Work out the finished part from the listing and answer in its coordinate system (mm). A direction names the side the tool comes from. Coordinates: 2 decimals unless noted, no trailing zeros. Order: outer loops, then holes, each group sorted by start corner. A loop starts at its lowest first (then second) coordinate and runs counter-clockwise, first axis right, second up. Notation, with made-up numbers: (45.5, 63) -> (81.5, 63) arc R13 ccw to (81.5, 82) -> close; hole circle Ø3 at (10, 7). An arc over 180 degrees is marked (long way). Use one line per item in the form item = value.
Autodesk Inventor part; units mm, degrees
ref_plane "nut_XY" through (0, 0, 0) normal (1, 0, 0) x (0, 0, -1)
ref_plane "nut_YZ" through (0, 0, 0) normal (0, 0, -1) x (0, 1, 0)
ref_plane "nut_ZX" through (0, 0, 0) normal (0, 1, 0) x (1, 0, 0)
sketch "Sketch_2" plane through (0, 0, 0) normal (0, 0, 1) x (1, 0, 0)
  arc A0 (-4.1, -2.7438) -> (-3.972, -2.9896) centre (-3.8, -2.7438) ccw
  line L0 (-3.972, -2.9896) -> (-1.1589, -4.9588)
  arc A1 (-1.1589, -4.9588) -> (-0.8, -4.7719) centre (-1.0281, -4.7719) ccw
  line L1 (-0.8, -4.7719) -> (-0.8, -2.9)
  line L2 (-0.8, -2.9) -> (-0.2, -2.9)
  arc A2 (-0.2, -2.9) -> (0, -2.7) centre (-0.2, -2.7) ccw
  line L3 (0, -2.7) -> (0, 2.7)
  arc A3 (0, 2.7) -> (-0.2, 2.9) centre (-0.2, 2.7) ccw
  line L4 (-0.2, 2.9) -> (-0.8, 2.9)
  line L5 (-0.8, 2.9) -> (-0.8, 4.7719)
  arc A4 (-0.8, 4.7719) -> (-1.1589, 4.9588) centre (-1.0281, 4.7719) ccw
  line L6 (-1.1589, 4.9588) -> (-3.972, 2.9896)
  arc A5 (-3.972, 2.9896) -> (-4.1, 2.7438) centre (-3.8, 2.7438) ccw
  line L7 (-4.1, 2.7438) -> (-4.1, -2.7438)
extrude "Extrusion1" add sketch "Sketch_2" along normal mid plane 10
sketch "Sketch_5" plane through (0, 0, 0) normal (0, 0, 1) x (1, 0, 0)
  line L0 (0, 0) -> (-4.1, 0)
  line L1 (-4.1, 0) -> (-4.1, 2)
  line L2 (-4.1, 2) -> (-3.721, 1.621)
  line L3 (-3.721, 1.621) -> (-0.379, 1.621)
  line L4 (-0.379, 1.621) -> (0, 2)
  line L5 (0, 2) -> (0, 0)
  line L6 (0, 0) -> (-4.1, 0)
revolve "Revolution1" cut sketch "Sketch_5" angle 360 about axis through (0, 0, 0) along (1, 0, 0)
thread "Thread1"
ref_plane "nut_XY" through (0, 0, 0) normal (1, 0, 0) x (0, 0, -1)
ref_plane "nut_YZ" through (0, 0, 0) normal (0, 0, -1) x (0, 1, 0)
ref_plane "nut_ZX" through (0, 0, 0) normal (0, 1, 0) x (1, 0, 0)
ref_plane "to_bolt_XY" through (-4.1, 0, 0) normal (1, 0, 0) x (0, 0, -1)
ref_plane "to_bolt_YZ" through (-4.1, 0, 0) normal (0, 0, -1) x (0, 1, 0)
ref_plane "to_bolt_ZX" through (-4.1, 0, 0) normal (0, 1, 0) x (1, 0, 0)
ref_plane "to_frames_XY" through (-0.8, 0, 0) normal (1, 0, 0) x (0, 0, -1)
ref_plane "to_frames_YZ" through (-0.8, 0, 0) normal (0, 0, -1) x (0, 1, 0)
ref_plane "to_frames_ZX" through (-0.8, 0, 0) normal (0, 1, 0) x (1, 0, 0)
ref_plane "to_lane_XY" through (0, 0, 0) normal (0, 0, 1) x (1, 0, 0)
ref_plane "to_lane_YZ" through (0, 0, 0) normal (1, 0, 0) x (0, 1, 0)
ref_plane "to_lane_ZX" through (0, 0, 0) normal (0, 1, 0) x (0, 0, 1)
properties part number "HNTT5-4" material "알루미늄 6061"
(1) Which of the six approach directions +Z, -Z, +X, -X, +Y, -Y give full straight-line access (tool end or side, diameter ignored) to faces 1 (the flat face through (-2, 0, -5)), 2 (the flat face through (-0.8, 4, 0)), 3 (the flat face through (-0.8, -4, 0))?
Data:
face_1 = -Z, +X, -X, +Y, -Y
face_2 = +Z, -Z, +X, +Y
face_3 = +Z, -Z, +X, -Y
(2) Section B-B on y = 0 is taken. Write down the section's boundary in (x, z), plus the area to 3 significant figures.
Data:
outline = (-4.1, -5) -> (0, -5) -> (0, -2) -> (-0.38, -1.62) -> (-3.72, -1.62) -> (-4.1, -2) -> close; (-4.1, 2) -> (-3.72, 1.62) -> (-0.38, 1.62) -> (0, 2) -> (0, 5) -> (-4.1, 5) -> close
area = 27.4 mm²
(3) Section A-A on z = 0 is taken. Write down the section's boundary in (x, y).
Data:
outline = (-4.1, -2.74) arc R0.3 ccw to (-3.97, -2.99) -> (-1.16, -4.96) arc R0.23 ccw to (-0.8, -4.77) -> (-0.8, -2.9) -> (-0.2, -2.9) arc R0.2 ccw to (0, -2.7) -> (0, -2) -> (-0.38, -1.62) -> (-3.72, -1.62) -> (-4.1, -2) -> close; (-4.1, 2) -> (-3.72, 1.62) -> (-0.38, 1.62) -> (0, 2) -> (0, 2.7) arc R0.2 ccw to (-0.2, 2.9) -> (-0.8, 2.9) -> (-0.8, 4.77) arc R0.23 ccw to (-1.16, 4.96) -> (-3.97, 2.99) arc R0.3 ccw to (-4.1, 2.74) -> close
(4) Each of these flat-tipped pins is pushed along its axis until it touches: P1, Ø0.9, axis at y = -3.5, z = -1.5, coming from the +X side; P2, Ø4, axis at y = 3.5, z = -0.5, coming from the -X side. Where does it stop, or does it pass through?
Data:
P1 = -0.8
P2 = -4.1
(5) Section D-D on z = 4.25 is taken. Write down the section's boundary in (x, y), plus the area to 3 significant figures.
Data:
outline = (-4.1, -2.74) arc R0.3 ccw to (-3.97, -2.99) -> (-1.16, -4.96) arc R0.23 ccw to (-0.8, -4.77) -> (-0.8, -2.9) -> (-0.2, -2.9) arc R0.2 ccw to (0, -2.7) -> (0, 2.7) arc R0.2 ccw to (-0.2, 2.9) -> (-0.8, 2.9) -> (-0.8, 4.77) arc R0.23 ccw to (-1.16, 4.96) -> (-3.97, 2.99) arc R0.3 ccw to (-4.1, 2.74) -> close
area = 31.3 mm²
(6) The mould has two halves that part along Z. Classify faces 4 (the cylindrical face through (-2.027, 0.748, -1.438)), 5 (the flat face through (-2.546, 3.988, -0.07)), 6 (the flat face through (-2, 0, 5)): released by +Z, released by -Z, zero draft, split by the parting line, or undercut.
Data:
face_4 = undercut
face_5 = zero draft
face_6 = released by +Z
(7) Straight lines are drawn through the part: line 1 along Z through (x, y) = (-1.1, 0); line 2 along Y through (x, z) = (-0.35, -3); line 3 along X through (y, z) = (1.5, 1). For each, find the intervals that lie inside material, in ascending order.
Data:
line_1 = -5 to -1.62, 1.62 to 5
line_2 = -2.9 to 2.9
line_3 = -3.9 to -0.2
(8) Section C-C on x = -3.1 is taken. Write down the section's boundary in (y, z), plus the area to 3 significant figures.
Data:
outline = (-3.6, -5) -> (3.6, -5) -> (3.6, 5) -> (-3.6, 5) -> close; hole circle Ø3.24 at (0, 0)
area = 63.7 mm²
